from build123d import *

# Parameters (mm, degrees)
F0_W     = 30
F0_H     = 160
F1_DEPTH = 3
F2_R     = 11
F3_DEPTH = 25
F4_R     = 11
F5_DEPTH = 25
F6_R     = 14.485281
F7_R     = 14.485281


with BuildPart() as f1:
    # F0 (on Top) → F1 (new body)
    with BuildSketch(Plane.XY):
        Rectangle(F0_W, F0_H)
    extrude(amount=F1_DEPTH)

    # F2 (on face) → F3 (cut)
    with BuildSketch(Plane.XY.offset(3)):
        Circle(F2_R)
    extrude(amount=-F3_DEPTH, mode=Mode.SUBTRACT)

    # F4 (on Top) → F5 (cut)
    with BuildSketch(Plane.XY):
        with Locations((0, 60)):
            Circle(F4_R)
        with Locations((0, -60)):
            Circle(F4_R)
    extrude(amount=F5_DEPTH, mode=Mode.SUBTRACT)

    # F6
    f6_edges = [f1.edges().sort_by_distance(p)[0] for p in [
        (-15, -80, 1.5),
        (15, -80, 1.5),
    ]]
    fillet(f6_edges, radius=F6_R)

    # F7
    f7_edges = [f1.edges().sort_by_distance(p)[0] for p in [
        (-15, 80, 1.5),
        (15, 80, 1.5),
    ]]
    fillet(f7_edges, radius=F7_R)


solid = f1.part
Can you work these out from the model? Positions are in its coordinate system, mm. Coordinates: 2 decimals unless noted, no trailing zeros. Order: outer loops, then holes, each group sorted by start corner. A loop starts at its lowest first (then second) coordinate and runs counter-clockwise, first axis right, second up. Notation, with made-up numbers: (-5.5, -39) - (25.5, -39) arc R12 cw to (25.5, -20) - close; hole circle Ø1 at (70, 55). An arc over 180 degrees is marked (long way). Answer as a JSON object with one key per item and string values. Group by question number.
Q1. Imagine slicing it at B-B (x = -7). Please give me the cut outline in (y, z).
Q2. We'd pull the mould along X, two halves only. Please class faces 1 (the face through (-1.432, 70.906, 1.479)), 2 (the face through (10.644, 75.869, 1.521)), 3 (the face through (-1.432, -49.094, 1.479)), 4 (the face through (-10.869, 75.644, 1.521)): +X half, -X half, draft (parallel to the pull), parting line (faces both ways), or undercut.
Q3. Imagine slicing it at C-C (z = 0.6). Please give me the cut outline in (x, y).
Q4. Imagine slicing it at D-D (x = 6). Please give me the cut outline in (y, z).
Q5. I need wall thicknesses on line 1 (Y direction, x = 0, z = 0.75); line 2 (X direction, y = 60, z = 0.9); line 3 (Y direction, x = 2.5, z = 2.45). Which ranges of each line are inside material? Lowest first, please. Write a range as from..to.
Q6. Imagine slicing it at A-A (y = 0). Please give me the cut outline in (x, z), and give its area (3 significant figures).
Q7. Will these pins go through, and if not, where does the flat tip stop? P1, Ø1, axis at x = 1, z = 1.5, coming from the +Y side; P2, Ø1, axis at x = -10.5, z = 2.5, coming from the +Y side.
Determined:
{
 "1": {"outline": "(-78.47, 0) - (-68.49, 0) - (-68.49, 3) - (-78.47, 3) - close; (-51.51, 0) - (-8.49, 0) - (-8.49, 3) - (-51.51, 3) - close; (8.49, 0) - (51.51, 0) - (51.51, 3) - (8.49, 3) - close; (68.49, 0) - (78.47, 0) - (78.47, 3) - (68.49, 3) - close"},
 "2": {"face 1": "undercut", "face 2": "+X half", "face 3": "undercut", "face 4": "-X half"},
 "3": {"outline": "(-15, -65.51) arc R14.49 ccw to (-0.51, -80) - (0.51, -80) arc R14.49 ccw to (15, -65.51) - (15, 65.51) arc R14.49 ccw to (0.51, 80) - (-0.51, 80) arc R14.49 ccw to (-15, 65.51) - close; hole circle Ø22 at (0, -60); hole circle Ø22 at (0, 0); hole circle Ø22 at (0, 60)"},
 "4": {"outline": "(-78.92, 0) - (-69.22, 0) - (-69.22, 3) - (-78.92, 3) - close; (-50.78, 0) - (-9.22, 0) - (-9.22, 3) - (-50.78, 3) - close; (9.22, 0) - (50.78, 0) - (50.78, 3) - (9.22, 3) - close; (69.22, 0) - (78.92, 0) - (78.92, 3) - (69.22, 3) - close"},
 "5": {"line 1": "y = -80..-71, -49..-11, 11..49, 71..80", "line 2": "x = -15..-11, 11..15", "line 3": "y = -79.86..-70.71, -49.29..-10.71, 10.71..49.29, 70.71..79.86"},
 "6": {"outline": "(-15, 0) - (-11, 0) - (-11, 3) - (-15, 3) - close; (11, 0) - (15, 0) - (15, 3) - (11, 3) - close", "area": "24.0 mm2"},
 "7": {"P1": "stops at y = 80", "P2": "stops at y = 76.46"}
}
